Could you check a few things on this model? Use its own coordinates, in mm. A direction names the side the tool comes from. Round coordinates to 2 decimals unless told otherwise and drop trailing zeros. Write each loop counter-clockwise with the first axis right and the second up, starting at its lowest first coordinate (ties: lowest second). Pieces come first, ordered by that corner, then holes. Notation, with made-up numbers: (76, 54.5) -> (131, 54.5) arc R19 cw to (131, 74.5) -> close; hole circle Ø6 at (17, 2.5). An arc over 180 degrees is marked (long way). Answer in a Markdown table with one row per item. Add a question column.
```python
from build123d import *

# Parameters (mm, degrees)
BOSS_EXTRUDE1_DEPTH = 14
BOSS_EXTRUDE2_START = 2
BOSS_EXTRUDE2_DEPTH = 2
SKETCH4_W           = 2
SKETCH4_H           = 12
CUT_EXTRUDE1_DEPTH  = 94
SKETCH5_R           = 1.7
SKETCH5_R_2         = 18
CUT_EXTRUDE2_DEPTH  = 10
CUT_EXTRUDE3_DEPTH  = 1


with BuildPart() as part:
    # Sketch1 → Boss-Extrude1 (new body)
    with BuildSketch(Plane.XY):
        with BuildLine():
            Line((52, 47.45), (-52, 47.45))
            ThreePointArc((-52, 47.45), (-55.853731957, 45.853731957), (-57.45, 42))
            Line((-57.45, 42), (-57.45, -42))
            ThreePointArc((-57.45, -42), (-55.853731957, -45.853731957), (-52, -47.45))
            Line((-52, -47.45), (52, -47.45))
            ThreePointArc((52, -47.45), (55.853731957, -45.853731957), (57.45, -42))
            Line((57.45, -42), (57.45, 42))
            ThreePointArc((57.45, 42), (55.853731957, 45.853731957), (52, 47.45))
        make_face()
        with BuildLine():
            Line((52, 45.45), (-52, 45.45))
            ThreePointArc((-52, 45.45), (-54.439518395, 44.439518395), (-55.45, 42))
            Line((-55.45, 42), (-55.45, -42))
            ThreePointArc((-55.45, -42), (-54.439518395, -44.439518395), (-52, -45.45))
            Line((-52, -45.45), (52, -45.45))
            ThreePointArc((52, -45.45), (54.439518395, -44.439518395), (55.45, -42))
            Line((55.45, -42), (55.45, 42))
            ThreePointArc((55.45, 42), (54.439518395, 44.439518395), (52, 45.45))
        make_face(mode=Mode.SUBTRACT)
    extrude(amount=BOSS_EXTRUDE1_DEPTH)

    # Sketch2 → Boss-Extrude2 (add)
    with BuildSketch(Plane(origin=(0, 0, 0), x_dir=(-1, 0, 0), z_dir=(0, 0, -1)).offset(BOSS_EXTRUDE2_START)):
        with BuildLine():
            Line((-57.45, 42), (-57.45, -42))
            ThreePointArc((-57.45, -42), (-55.853731957, -45.853731957), (-52, -47.45))
            Line((-52, -47.45), (52, -47.45))
            ThreePointArc((52, -47.45), (55.853731957, -45.853731957), (57.45, -42))
            Line((57.45, -42), (57.45, 42))
            ThreePointArc((57.45, 42), (55.853731957, 45.853731957), (52, 47.45))
            Line((52, 47.45), (-52, 47.45))
            ThreePointArc((-52, 47.45), (-55.853731957, 45.853731957), (-57.45, 42))
        make_face()
    extrude(amount=-BOSS_EXTRUDE2_DEPTH)

    # Sketch4 → Cut-Extrude1 (cut)
    with BuildSketch(Plane.XY):
        Polygon((-4.554445608, 45.9), (-4.554445608, 47.45), (-20.554445608, 47.45), (-20.554445608, 45.45), (-4.554445608, 45.45), align=None)
        with Locations((-56.45, 0.205355748)):
            Rectangle(SKETCH4_W, SKETCH4_H)
        Polygon((55.445554392, -35.534861573), (57.45, -35.534861573), (57.45, -17.740217321), (55.45, -17.740217321), align=None)
    extrude(amount=CUT_EXTRUDE1_DEPTH, mode=Mode.SUBTRACT)

    # Sketch5 → Cut-Extrude2 (cut)
    with BuildSketch(Plane(origin=(0, 0, -2), x_dir=(-1, 0, 0), z_dir=(0, 0, -1))):
        with Locations((-14.281468852, 16)):
            Circle(SKETCH5_R)
        with Locations((-46.281468852, 16)):
            Circle(SKETCH5_R)
        with Locations((-46.281468852, -16)):
            Circle(SKETCH5_R)
        with Locations((-14.281468852, -16)):
            Circle(SKETCH5_R)
        with Locations((-30.281468852, 0)):
            Circle(SKETCH5_R_2)
    extrude(amount=-CUT_EXTRUDE2_DEPTH, mode=Mode.SUBTRACT)

    # Sketch6 → Cut-Extrude3 (cut)
    with BuildSketch(Plane(origin=(0, 0, -2), x_dir=(-1, 0, 0), z_dir=(0, 0, -1))):
        Polygon((25.401519513, 0), (20.78271736, 0), (30.173596476, -16.265479758), (39.564475593, 0), (34.945673439, 0), (30.173596476, -8.265479758), align=None)
        Polygon((24.070013842, 3.906235473), (26.325279944, 0), (26.433549893, 0), (33.901298637, 12.934520242), (29.282496484, 12.934520242), align=None)
        Polygon((-2.587238376, 17.734520242), (7.65179166, 0), (12.270593814, 0), (4.340964855, 13.734520242), (11.92932797, 13.734520242), (9.619926893, 17.734520242), align=None)
        Polygon((12.270593814, 0), (7.65179166, 0), (17.042670777, -16.265479758), (23.146253411, -5.693764527), (20.836852334, -1.693764527), (17.042670777, -8.265479758), align=None)
        Polygon((10.543687324, 17.734520242), (20.78271736, 0), (25.401519513, 0), (17.471890554, 13.734520242), (29.744376699, 13.734520242), (42.875302398, 13.734520242), (34.945673439, 0), (39.564475593, 0), (49.803505629, 17.734520242), (36.672579929, 17.734520242), align=None)
    extrude(amount=-CUT_EXTRUDE3_DEPTH, mode=Mode.SUBTRACT)


solid = part.part
```
(1) If we mould it in two halves opening along X, with no side actions, what happens to faces 1 (the face through (-36, 1, -1)), 2 (the face through (55.811, 45.896, 5.888)), 3 (the face through (-55.896, 45.811, 5.888))? For each: pulls with the +X half, pulls with the -X half, needs draft (parallel to the pull), parting line crosses it, or undercut.
(2) For P1, Ø7, axis at y = -23.5, z = 6, coming from the +X side; P2, Ø2, axis at x = 9.5, y = -31.5, coming from the +Z side; P3, Ø0.6, axis at x = -56, z = 7, coming from the -Y side; P4, Ø4.5, axis at x = 46.28, y = -16, coming from the -Z side, each with a flat end and sliding along its axis, tell me the tip position at first contact or that it passes through.
(3) Suppose I cut it at A-A, the plane z = 12.25. Please give me the cut outline in (x, y), then the cut area to 3 significant figures.
(4) Suppose I cut it at C-C, the plane y = 39. Please give me the cut outline in (x, z), then the cut area to 3 significant figures.
(5) On a 3-axis mill with a long thin cutter (end or side, diameter ignored), from which of +Z, -Z, +X, -X, +Y, -Y can I reach the whole of each face in a straight line? I mean faces 4 (the face through (56, 29, 14)), 5 (the face through (-20.052, -11.054, -1.507)), 6 (the face through (-55.45, 24, 7)). Say none if no direction works.
(6) Suppose I cut it at D-D, the plane y = 16. Please give me the cut outline in (x, z).
(7) I need wall thicknesses on L1, parallel to Y at x = -38, z = 9.5; L2, parallel to X at y = 37, z = 0.75; L3, parallel to Z at x = -51, y = 16.5. Which ranges of each line are inside material? Lowest first, please.
(8) Suppose I cut it at B-B, the plane y = 2. Please give me the cut outline in (x, z).
Response:
| question | item | result |
|---|---|---|
| 1 | face 1 | undercut |
| 1 | face 2 | pulls with the +X half |
| 1 | face 3 | pulls with the -X half |
| 2 | P1 | x = -55.45 |
| 2 | P2 | z = 0 |
| 2 | P3 | y = -46 |
| 2 | P4 | z = -2 |
| 3 | outline | (-57.45, -42) arc R5.45 ccw to (-52, -47.45) -> (52, -47.45) arc R5.45 ccw to (57.45, -42) -> (57.45, -35.53) -> (55.45, -35.53) -> (55.45, -42) arc R3.45 cw to (52, -45.45) -> (-52, -45.45) arc R3.45 cw to (-55.45, -42) -> (-55.45, -5.79) -> (-57.45, -5.79) -> close; (-57.45, 6.21) -> (-55.45, 6.21) -> (-55.45, 42) arc R3.45 cw to (-52, 45.45) -> (-20.55, 45.45) -> (-20.55, 47.45) -> (-52, 47.45) arc R5.45 ccw to (-57.45, 42) -> close; (-4.55, 45.45) -> (52, 45.45) arc R3.45 cw to (55.45, 42) -> (55.45, -17.74) -> (57.45, -17.74) -> (57.45, 42) arc R5.45 ccw to (52, 47.45) -> (-4.55, 47.45) -> close |
| 3 | area | 716 mm² |
| 4 | outline | (-57.45, -2) -> (57.45, -2) -> (57.45, 14) -> (55.45, 14) -> (55.45, 0) -> (-55.45, 0) -> (-55.45, 14) -> (-57.45, 14) -> close |
| 4 | area | 286 mm² |
| 5 | face 4 | +Z, +X, -X, +Y, -Y |
| 5 | face 5 | -Z |
| 5 | face 6 | +Z |
| 6 | outline | (-57.45, -2) -> (-48.8, -2) -> (-48.8, -1) -> (-11.55, -1) -> (-11.55, -2) -> (-10.62, -2) -> (-10.62, -1) -> (1.59, -1) -> (1.59, -2) -> (12.58, -2) -> (12.58, 0) -> (-55.45, 0) -> (-55.45, 14) -> (-57.45, 14) -> close; (15.98, -2) -> (22.04, -2) -> (22.04, 0) -> (15.98, 0) -> close; (38.53, -2) -> (44.58, -2) -> (44.58, 0) -> (38.53, 0) -> close; (47.98, -2) -> (57.45, -2) -> (57.45, 14) -> (55.45, 14) -> (55.45, 0) -> (47.98, 0) -> close |
| 7 | L1 | -47.45 to -45.45, 45.45 to 47.45 |
| 7 | L2 | -57.45 to -55.45, 55.45 to 57.45 |
| 7 | L3 | -2 to 0 |
| 8 | outline | (-57.45, -2) -> (-40.72, -2) -> (-40.72, -1) -> (-36.1, -1) -> (-36.1, -2) -> (-27.59, -2) -> (-27.59, -1) -> (-25.17, -1) -> (-25.17, -2) -> (-24.25, -2) -> (-24.25, -1) -> (-19.63, -1) -> (-19.63, -2) -> (-11.12, -2) -> (-11.12, -1) -> (-6.5, -1) -> (-6.5, -2) -> (12.39, -2) -> (12.39, 0) -> (-57.45, 0) -> close; (48.17, -2) -> (57.45, -2) -> (57.45, 14) -> (55.45, 14) -> (55.45, 0) -> (48.17, 0) -> close |
